Could you check a few things on this model? Use its own coordinates, in mm. A direction names the side the tool comes from. Give positions to 0.01 mm unless a question says otherwise; leave off trailing zeros. Loops run counter-clockwise (first coordinate to the right, second up) from the corner with the lowest first, then second, coordinate; pieces in that order, holes last. Notation, with made-up numbers: (-15.5, 81) - (-7.5, 81) arc R19 ccw to (-7.5, 86) - close; hole circle Ø4 at (-26.75, 34.5). An arc over 180 degrees is marked (long way). Answer in a Markdown table with one row per item. Add a question column.
```python
from build123d import *

# Parameters (mm, degrees)
BOSS_EXTRUDE1_DEPTH = 254
SKETCH2_W           = 1219.2
SKETCH2_H           = 1193.8
BOSS_EXTRUDE2_DEPTH = 12.7
SKETCH3_W           = 25.4
SKETCH3_H           = 44.45
BOSS_EXTRUDE3_DEPTH = 254


with BuildPart() as part:
    # Sketch1 → Boss-Extrude1 (new body)
    with BuildSketch(Plane(origin=(0, 0, 0), x_dir=(1, 0, 0), z_dir=(0, 1, 0))):
        Polygon((-596.9, -584.2), (-596.9, 584.2), (596.9, 584.2), (596.9, -584.2), (596.9, -596.9), (609.6, -596.9), (609.6, 596.9), (-609.6, 596.9), (-609.6, -596.9), (-596.9, -596.9), align=None)
    extrude(amount=BOSS_EXTRUDE1_DEPTH)

    # Sketch2 → Boss-Extrude2 (add)
    with BuildSketch(Plane.XZ):
        Rectangle(SKETCH2_W, SKETCH2_H)
    extrude(amount=BOSS_EXTRUDE2_DEPTH)

    # Sketch3 → Boss-Extrude3 (add)
    with BuildSketch(Plane(origin=(0, 0, 0), x_dir=(1, 0, 0), z_dir=(0, 1, 0))):
        with Locations((-584.2, 561.975)):
            Rectangle(SKETCH3_W, SKETCH3_H)
        with Locations((584.2, 561.975)):
            Rectangle(SKETCH3_W, SKETCH3_H)
    extrude(amount=BOSS_EXTRUDE3_DEPTH)


solid = part.part
```
(1) For pin 1 Ø12 at (x, y) = (-314.5, 118.5) entering from +Z; pin 2 Ø8 at (x, z) = (241.5, -139.5) entering from +Y; pin 3 Ø12.5 at (x, y) = (-583, 68.5) entering from +Z, each with a flat end and sliding along its axis, tell me the tip position at first contact or that it passes through.
(2) We'd pull the mould along X, two halves only. Please class faces 3 (the flat face through (571.5, 125, -562)), 4 (the flat face through (-596.9, 125, 37)), 5 (the flat face through (-9, 123, -596.9)), 6 (the flat face through (609.6, 123, -8)): pulls with the +X half, pulls with the -X half, needs draft (parallel to the pull), parting line crosses it, or undercut.
(3) I want a section at B-B on x = -129. Please give me the cut outline in (y, z), then the cut area to 3 significant figures.
(4) I want a section at C-C on z = 75. Please give me the cut outline in (x, y), then the cut area to 3 significant figures.
(5) Please list where these lines run through material, in increasing order: line 1 (X direction, y = 42.5, z = -214); line 2 (Z direction, x = 474, y = 145); line 3 (Y direction, x = 7.5, z = -273).
(6) On a 3-axis mill with a long thin cutter (end or side, diameter ignored), from which of +Z, -Z, +X, -X, +Y, -Y can I reach the whole of each face in a straight line? I mean faces 1 (the flat face through (596.9, 125, 21)), 2 (the flat face through (-9, -12.7, 8)). Say none if no direction works.
(7) I want a section at A-A on y = 28. Please give me the cut outline in (x, z).
Reported:
| question | item | result |
|---|---|---|
| 1 | pin 1 | z = -584.2 |
| 1 | pin 2 | y = 0 |
| 1 | pin 3 | z = -539.75 |
| 2 | face 3 | undercut |
| 2 | face 4 | undercut |
| 2 | face 5 | needs draft |
| 2 | face 6 | pulls with the +X half |
| 3 | outline | (-12.7, -596.9) - (254, -596.9) - (254, -584.2) - (0, -584.2) - (0, 596.9) - (-12.7, 596.9) - close |
| 3 | area | 18,400 mm² |
| 4 | outline | (-609.6, -12.7) - (609.6, -12.7) - (609.6, 254) - (596.9, 254) - (596.9, 0) - (-596.9, 0) - (-596.9, 254) - (-609.6, 254) - close |
| 4 | area | 21,900 mm² |
| 5 | line 1 | -609.6 to -596.9, 596.9 to 609.6 |
| 5 | line 2 | -596.9 to -584.2 |
| 5 | line 3 | -12.7 to 0 |
| 6 | face 1 | +Z, +Y |
| 6 | face 2 | +Z, -Z, +X, -X, -Y |
| 7 | outline | (-609.6, -596.9) - (609.6, -596.9) - (609.6, 596.9) - (596.9, 596.9) - (596.9, -539.75) - (571.5, -539.75) - (571.5, -584.2) - (-571.5, -584.2) - (-571.5, -539.75) - (-596.9, -539.75) - (-596.9, 596.9) - (-609.6, 596.9) - close |
